from build123d import *

# Parameters (mm, degrees)
PROFILES_R                  = 12
PROFILE_DEPTH               = 3
CONNECTINGWALLS_R           = 9.5
CONNECTINGWALLS_R_2         = 8.5
CONNECTINGWALL_DEPTH        = 5
CONNECTORCUTS_W             = 7
CONNECTORCUTS_H             = 4
CONNECTORCUT_DEPTH          = 19.761663039
CONNECTOR_REACH             = 20.762
CONNECTOR_DIRECTION_2_REACH = 20.762


with BuildPart() as part:
    # ProfileS → Profile (new body)
    with BuildSketch(Plane(origin=(0, 0, 0), x_dir=(1, 0, 0), z_dir=(0, 1, 0))):
        with Locations(Location((0, 0, 0), (0, 0, 270))):
            Circle(PROFILES_R)
    extrude(amount=PROFILE_DEPTH)

    # ConnectingWallS → ConnectingWall (add)
    with BuildSketch(Plane(origin=(0, 3, 0), x_dir=(1, 0, 0), z_dir=(0, 1, 0))):
        with Locations(Location((0, 0, 0), (0, 0, 270))):
            Circle(CONNECTINGWALLS_R)
        with Locations(Location((0, 0, 0), (0, 0, 270))):
            Circle(CONNECTINGWALLS_R_2, mode=Mode.SUBTRACT)
    extrude(amount=CONNECTINGWALL_DEPTH)

    # ConnectorCutS → ConnectorCut (cut, through all)
    with BuildSketch(Plane.XZ):
        Rectangle(CONNECTORCUTS_W, CONNECTORCUTS_H)
    extrude(amount=-CONNECTORCUT_DEPTH, mode=Mode.SUBTRACT)

    # Connector: up to this face of the body (flat: up to its plane)
    connector_end = Plane(part.part.faces().sort_by_distance((0, 1.5, 2))[0])
    # ConnectorS → Connector (add, up to the picked face)
    with BuildSketch(Plane.XY, mode=Mode.PRIVATE) as connector_sk1:
        Polygon((-3.5, 0), (-3.35, -3), (3.35, -3), (3.5, 0), (4.9, 0), (4.65, -5), (-4.65, -5), (-4.9, 0), align=None)
    connector_tool1 = split(extrude(connector_sk1.sketch, amount=CONNECTOR_REACH, mode=Mode.PRIVATE), bisect_by=connector_end, keep=Keep.BOTH, mode=Mode.PRIVATE)
    add(connector_tool1.solids().sort_by(Axis((0, -3.22549, 0), (0, 0, 1)))[0])

    # Connector direction 2: up to this face of the body (flat: up to its plane)
    connector_direction_2_end = Plane(part.part.faces().sort_by_distance((0, 1.5, -2))[0])
    # ConnectorS → Connector direction 2 (add, up to the picked face)
    with BuildSketch(Plane.XY, mode=Mode.PRIVATE) as connector_direction_2_sk1:
        Polygon((-3.5, 0), (-3.35, -3), (3.35, -3), (3.5, 0), (4.9, 0), (4.65, -5), (-4.65, -5), (-4.9, 0), align=None)
    connector_direction_2_tool1 = split(extrude(connector_direction_2_sk1.sketch, amount=-CONNECTOR_DIRECTION_2_REACH, mode=Mode.PRIVATE), bisect_by=connector_direction_2_end, keep=Keep.BOTH, mode=Mode.PRIVATE)
    add(connector_direction_2_tool1.solids().sort_by(Axis((0, -3.22549, 0), (0, 0, -1)))[0])


solid = part.part
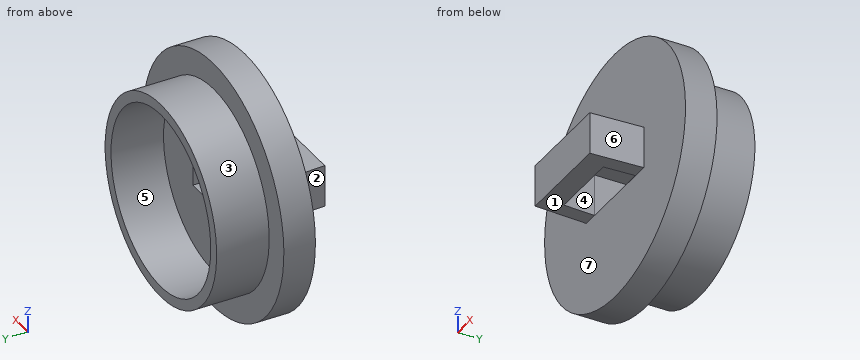
Design review of the part built by this model. Coordinates are the model's own, in mm. Face numbers are marked on the shaded views. A direction names the side the tool comes from. Coordinates: 2 decimals unless noted, no trailing zeros. Loops run counter-clockwise (first coordinate to the right, second up) from the corner with the lowest first, then second, coordinate; pieces in that order, holes last. Notation, with made-up numbers: M 41.25,51 L 55.25,51 A22 cw 55.25,86 Z; hole C -21,-33 d4. An arc over 180 degrees is marked long. Answer as CSV lines item,"result".
Item 1: The part is to be moulded in two halves that separate along X. For the marked faces 4, 5, 6 and 7, say which applies: pulls with the +X half, pulls with the -X half, needs draft (parallel to the pull), parting line crosses it, or undercut.
Answer list:
face 4,"undercut"
face 5,"undercut"
face 6,"pulls with the +X half"
face 7,"needs draft"
Item 2: Add section D-D on y = -0.5. State the section outline as (x, z) points (3 decimals).
Answer list:
outline,"M -4.875,-2 L -3.475,-2 L -3.475,2 L -4.875,2 Z; M 3.475,-2 L 4.875,-2 L 4.875,2 L 3.475,2 Z"
Item 3: For probe 1 along X at (y, z) = (5.35, 0); probe 2 along Z at (x, y) = (7.75, 6); probe 3 along Y at (x, z) = (-4.5, -2.75), list the stretches that pass through material, from the lowest coordinate up.
Answer list:
probe 1,"-9.5 to -8.5, 8.5 to 9.5"
probe 2,"-5.49 to -3.49, 3.49 to 5.49"
probe 3,"0 to 3"
Item 4: Add section A-A on x = 0.5. State the section outline as (y, z) points, plus the area to 3 significant figures.
Answer list:
outline,"M -5,-2 L -3,-2 L -3,2 L -5,2 Z; M 0,-11.99 L 3,-11.99 L 3,-9.49 L 8,-9.49 L 8,-8.49 L 3,-8.49 L 3,-2 L 0,-2 Z; M 0,2 L 3,2 L 3,8.49 L 8,8.49 L 8,9.49 L 3,9.49 L 3,11.99 L 0,11.99 Z"
area,"78.0 mm²"
Item 5: Add section C-C on y = 1.25. State the section outline as (x, z) points.
Answer list:
outline,"C 0,0 d24; hole M -3.5,-2 L 3.5,-2 L 3.5,2 L -3.5,2 Z"
Item 6: For P1, Ø1.5, axis at x = 1, y = 1, coming from the -Z side; P2, Ø0.9, axis at y = 1, z = -1, coming from the -X side; P3, Ø1.5, axis at x = -2.5, y = -3, coming from the +Z side, all flat-tipped, find the tip position at first contact; note any pin that passes through.
Answer list:
P1,"z = -12"
P2,"x = -11.99"
P3,"z = 2"
Item 7: Add section B-B on z = 0. State the section outline as (x, y) points.
Answer list:
outline,"M -12,0 L -4.9,0 L -4.65,-5 L 4.65,-5 L 4.9,0 L 12,0 L 12,3 L 9.5,3 L 9.5,8 L 8.5,8 L 8.5,3 L 3.5,3 L 3.5,0 L 3.35,-3 L -3.35,-3 L -3.5,0 L -3.5,3 L -8.5,3 L -8.5,8 L -9.5,8 L -9.5,3 L -12,3 Z"
Item 8: Machinability: for the marked faces 1, 2 and 3, which of the approach directions +Z, -Z, +X, -X, +Y, -Y give a long, thin tool a straight path to every point of the face, cutting with its end or side? Answer none if there is none.
Answer list:
face 1,"-Z, +X, -X, -Y"
face 2,"+Z, -Z, -X, -Y"
face 3,"+Y"
